```python
from build123d import *

# Parameters (mm, degrees)
SKETCH_2_R          = 5
EXTRUDE_1_DEPTH     = 3
CUT_EXTRUDE_1_DEPTH = 200.932491601


with BuildPart() as part:
    # Sketch 2 → Extrude 1 (new body)
    # profile 1 of 2: a face of its own
    with BuildSketch(Plane(origin=(0, 0, 0), x_dir=(1, 0, 0), z_dir=(0, 1, 0))):
        with BuildLine():
            Line((-158, 4.647580015), (-158, -4.647580015))
            add(Edge.make_bspline(
                [(-158, -4.647580015), (-157.840632623, -7.898309914), (-157.230923207, -14.322386142), (-155.452746954, -23.836708418), (-151.455463066, -36.074052553), (-145.999672069, -47.671836442), (-139.230379225, -58.550935995), (-131.318807935, -68.627343709), (-120.682359228, -79.66101812), (-106.314153227, -91.393620751), (-87.729388125, -102.749099806), (-64.740966029, -112.518967886), (-39.976202938, -119.201809502), (-14.818936259, -122.590822364), (10.300366837, -122.846161773), (35.006186274, -120.076750254), (58.936571944, -114.347737623), (81.928105159, -105.552677383), (101.115324182, -94.89380247), (116.213750165, -83.595995995), (127.601010627, -72.704005397), (135.860607987, -63.075817152), (142.879120728, -52.984121912), (148.765002816, -42.186376352), (154.133853951, -28.8835882), (156.763243516, -17.891175579), (157.749742083, -9.75226901), (158, -4.647580015)],
                knots=[0, 0, 0, 0, 0, 0.030050103, 0.059543416, 0.089055708, 0.11857173, 0.148087684, 0.177604234, 0.207120827, 0.259849884, 0.318883484, 0.377917011, 0.436950613, 0.495984189, 0.552632218, 0.609280233, 0.665928258, 0.722576279, 0.779224237, 0.811190919, 0.839514883, 0.867838217, 0.896161221, 0.924483933, 0.952811697, 1, 1, 1, 1, 1], degree=4))
            Line((158, -4.647580015), (158, 4.647580015))
            add(Edge.make_bspline(
                [(-158, 4.647580015), (-157.840632623, 7.898309914), (-157.230923207, 14.322386142), (-155.452746954, 23.836708418), (-151.455463066, 36.074052553), (-145.999672069, 47.671836442), (-139.230379225, 58.550935995), (-131.318807935, 68.627343709), (-120.682359228, 79.66101812), (-106.314153227, 91.393620751), (-87.729388125, 102.749099806), (-64.740966029, 112.518967886), (-39.976202938, 119.201809502), (-14.818936259, 122.590822364), (10.300366837, 122.846161773), (35.006186274, 120.076750254), (58.936571944, 114.347737623), (81.928105159, 105.552677383), (101.115324182, 94.89380247), (116.213750165, 83.595995995), (127.601010627, 72.704005397), (135.860607987, 63.075817152), (142.879120728, 52.984121912), (148.765002816, 42.186376352), (154.133853951, 28.8835882), (156.763243516, 17.891175579), (157.749742083, 9.75226901), (158, 4.647580015)],
                knots=[0, 0, 0, 0, 0, 0.030050103, 0.059543416, 0.089055708, 0.11857173, 0.148087684, 0.177604234, 0.207120827, 0.259849884, 0.318883484, 0.377917011, 0.436950613, 0.495984189, 0.552632218, 0.609280233, 0.665928258, 0.722576279, 0.779224237, 0.811190919, 0.839514883, 0.867838217, 0.896161221, 0.924483933, 0.952811697, 1, 1, 1, 1, 1], degree=4))
        make_face()
        with BuildLine():
            Line((128, 3.843082438), (128, -3.843082438))
            add(Edge.make_bspline(
                [(128, -3.843082438), (127.817421208, -6.922474495), (127.017736472, -13.034900149), (123.690358435, -25.137176558), (116.36700284, -39.700766823), (103.097371825, -55.45268215), (86.250252489, -68.789883395), (66.760356672, -79.331620625), (38.336266983, -89.434633735), (-1.8863e-05, -94.501089514), (-38.336499093, -89.434556711), (-66.760338924, -79.331638367), (-86.250604016, -68.789751516), (-103.097493512, -55.452466033), (-116.367130615, -39.700780131), (-123.690887414, -25.135387447), (-127.01753099, -13.035584443), (-127.817439146, -6.922588381), (-128, -3.843132274)],
                knots=[0.002244566, 0.002244566, 0.002244566, 0.002244566, 0.033354271, 0.064463976, 0.126683386, 0.188902797, 0.251122207, 0.313341617, 0.375561028, 0.499999848, 0.624438669, 0.68665808, 0.74887749, 0.8110969, 0.873316311, 0.935535721, 0.966645426, 0.997755131, 0.997755131, 0.997755131, 0.997755131], degree=3))
            Line((-128, -3.843132274), (-128, 3.843132274))
            add(Edge.make_bspline(
                [(-128, 3.843132274), (-127.817439146, 6.922588381), (-127.01753099, 13.035584443), (-123.690887414, 25.135387447), (-116.367130615, 39.700780131), (-103.097493512, 55.452466033), (-86.250604016, 68.789751516), (-66.760338924, 79.331638367), (-38.336499093, 89.434556711), (-1.8863e-05, 94.501089514), (38.336266983, 89.434633735), (66.760356672, 79.331620625), (86.250252489, 68.789883395), (103.097371825, 55.45268215), (116.36700284, 39.700766823), (123.690358435, 25.137176558), (127.017736472, 13.034900149), (127.817421208, 6.922474495), (128, 3.843082438)],
                knots=[0.002244566, 0.002244566, 0.002244566, 0.002244566, 0.033354271, 0.064463976, 0.126683386, 0.188902797, 0.251122207, 0.313341617, 0.375561028, 0.499999848, 0.624438669, 0.68665808, 0.74887749, 0.8110969, 0.873316311, 0.935535721, 0.966645426, 0.997755131, 0.997755131, 0.997755131, 0.997755131], degree=3))
        make_face(mode=Mode.SUBTRACT)
    # profile 2 of 2: a face of its own
    with BuildSketch(Plane(origin=(0, 0, 0), x_dir=(1, 0, 0), z_dir=(0, 1, 0))):
        with BuildLine():
            Line((14.99999999, -91.826221469), (14.99999999, 91.826221469))
            add(Edge.make_bspline(
                [(-15, 91.826204624), (-10.017402995, 92.258274497), (-9.048e-06, 92.690700959), (10.017368309, 92.258290778), (14.99999999, 91.826221469)],
                knots=[0.459354839, 0.459354839, 0.459354839, 0.459354839, 0.499999848, 0.540645219, 0.540645219, 0.540645219, 0.540645219], degree=3))
            Line((-15, 91.826204625), (-15, -91.826204624))
            add(Edge.make_bspline(
                [(14.99999999, -91.826221469), (10.017368308, -92.258290778), (-9.048e-06, -92.690700959), (-10.017402995, -92.258274497), (-15, -91.826204624)],
                knots=[0.459354478, 0.459354478, 0.459354478, 0.459354478, 0.499999848, 0.540644858, 0.540644858, 0.540644858, 0.540644858], degree=3))
        make_face()
        with Locations(Location((0, 0, 0), (0, 0, 270))):
            Circle(SKETCH_2_R, mode=Mode.SUBTRACT)
    extrude(amount=EXTRUDE_1_DEPTH)

    # Sketch 3 → Cut-Extrude 1 (cut, through all)
    with BuildSketch(Plane(origin=(0, 3, 0), x_dir=(1, 0, 0), z_dir=(0, 1, 0))):
        Polygon((79.061701734, -95.271659003), (82.061668628, -95.257565394), (82.014689931, -85.257675744), (79.014723036, -85.271769353), align=None)
        Polygon((121.892616384, -59.179131978), (118.892649489, -59.193225587), (118.939628187, -69.193115237), (121.939595081, -69.179021627), align=None)
        Polygon((-0.858334219, -112.480728906), (2.141632676, -112.466635297), (2.094653978, -102.466745647), (-0.905312917, -102.480839257), align=None)
        Polygon((-37.87664199, -108.670646183), (-37.923620688, -98.670756533), (-40.923587583, -98.684850143), (-40.876608885, -108.684739792), align=None)
        Polygon((42.122475205, -108.294816603), (42.075496508, -98.294926953), (39.075529613, -98.309020563), (39.122508311, -108.308910212), align=None)
        Polygon((138.220248888, 2.149150661), (138.234342497, -0.850816234), (148.234232146, -0.803837537), (148.220138537, 2.196129358), align=None)
        Polygon((121.284233788, 70.321240537), (118.284266893, 70.307146928), (118.33124559, 60.307257278), (121.331212485, 60.321350887), align=None)
        Polygon((78.16307615, 96.009861114), (78.210054848, 86.009971464), (81.210021742, 86.024065074), (81.163043045, 96.023954723), align=None)
        Polygon((38.103152377, 108.671282743), (38.150131075, 98.671393094), (41.150097969, 98.685486703), (41.103119272, 108.685376352), align=None)
        Polygon((-1.868143592, 102.467382207), (1.131823303, 102.481475817), (1.084844606, 112.481365466), (-1.915122289, 112.467271857), align=None)
        Polygon((-41.895964819, 108.295453163), (-41.848986121, 98.295563514), (-38.849019226, 98.309657123), (-38.895997924, 108.309546772), align=None)
        Polygon((-81.835158242, 95.258201954), (-81.788179544, 85.258312304), (-78.788212649, 85.272405914), (-78.835191347, 95.272295563), align=None)
        Polygon((-118.7131178, 69.193751797), (-121.713084695, 69.179658188), (-121.666105997, 59.179768538), (-118.666139102, 59.193862147), align=None)
        Polygon((-148.00772176, 0.804474097), (-147.993628151, -2.195492798), (-137.993738501, -2.1485141), (-138.00783211, 0.851452795), align=None)
        Polygon((-118.104735204, -60.306620718), (-121.104702099, -60.320714327), (-121.057723401, -70.320603977), (-118.057756506, -70.306510367), align=None)
        Polygon((-80.936532658, -96.023318163), (-77.936565763, -96.009224554), (-77.983544461, -86.009334904), (-80.983511356, -86.023428513), align=None)
    extrude(amount=-CUT_EXTRUDE_1_DEPTH, mode=Mode.SUBTRACT)


solid = part.part
```
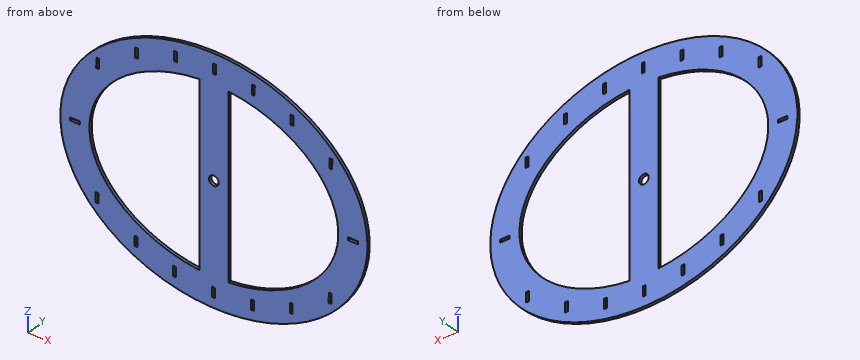
Part model, mm, in its own coordinate system. Coordinates: 2 decimals unless noted, no trailing zeros.
Item 1: Pin check, flat tips, straight feed: pin 1 (1.5 mm diameter, centred on y = 2, z = -15.5, fed in from +X); pin 2 (1.5 mm diameter, centred on x = -116, y = 1.5, fed in from +Z); pin 3 (1 mm diameter, centred on x = 118, y = 0.5, fed in from +Z). Stop position of each tip, or through.
Item 2: Slice it at A-A (y = 2.15). Count the separate pieces of the cut face and the enclosed holes in it, and give its area (3 significant figures).
Item 3: Probe line 1 (X direction, y = 1.35, z = 0); line 2 (X direction, y = 1.6, z = -20); line 3 (X direction, y = 1.75, z = 100). List the from-to ranges inside material, lowest first.
Results found:
1. pin 1: stops at x = 156.96
1. pin 2: stops at z = 83.85
1. pin 3: stops at z = 81.95
2. separate pieces: 1
2. enclosed holes: 19
2. area: 28,700 mm2
3. line 1: x = -158 to -148, -138 to -128, -15 to -5, 5 to 15, 128 to 138.23, 148.23 to 158
3. line 2: x = -155.99 to -125, -15 to 15, 125 to 155.99
3. line 3: x = -91.29 to -40.92, -37.92 to 39.08, 42.08 to 91.29
